from build123d import *

# Parameters (mm, degrees)
F1_DEPTH = 139.7
F2_R     = 6.731
F3_DEPTH = 25.4
F4_R     = 6.985
F5_DEPTH = 25.4
F6_R     = 1.27
F7_R     = 1.27


with BuildPart() as f1:
    # F0 (on Top) → F1 (new body)
    with BuildSketch(Plane.XY):
        Polygon((25.4, 0), (0, 9.525), (-25.4, 0), (0, -9.525), align=None)
    extrude(amount=F1_DEPTH)

    # F2 (on Top) → F3 (join)
    with BuildSketch(Plane.XY):
        Circle(F2_R)
    extrude(amount=-F3_DEPTH)

    # F4 (on face) → F5 (cut)
    with BuildSketch(Plane.XY.offset(139.7)):
        Circle(F4_R)
    extrude(amount=-F5_DEPTH, mode=Mode.SUBTRACT)

    # F6
    f6_edges = [f1.edges().sort_by_distance(p)[0] for p in [
        (-6.985, 0, 114.3),
        (-6.985, 0, 139.7),
    ]]
    fillet(f6_edges, radius=F6_R)

    # F7
    f7_edges = [f1.edges().sort_by_distance(p)[0] for p in [
        (-6.731, 0, -25.4),
        (-6.731, 0, 0),
    ]]
    fillet(f7_edges, radius=F7_R)


solid = f1.part
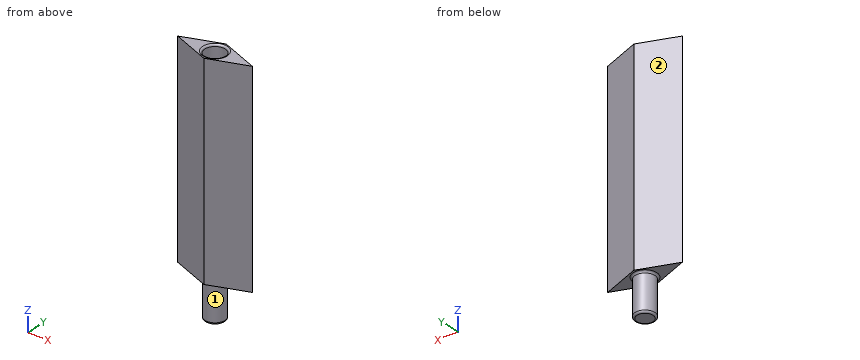
The listing builds one solid part. Answer for the finished solid, in the listing's coordinates (mm). Face numbers are marked on the shaded views. A direction names the side the tool comes from. Coordinates: 2 decimals unless noted, no trailing zeros. Write each loop counter-clockwise with the first axis right and the second up, starting at its lowest first coordinate (ties: lowest second). Pieces come first, ordered by that corner, then holes. Notation, with made-up numbers: (8, -38) - (27, -38) arc R36 ccw to (27, 0) - close; hole circle Ø4 at (11.5, 49.25). An arc over 180 degrees is marked (long way). Return JSON: item names as keys, results as strings.
1. Consider line 1 along Y through (x, z) = (0, 124) (3 decimals); line 2 along Z through (x, y) = (-1.5, 8.25); line 3 along Y through (x, z) = (13, 68). Determine where each line is inside the solid, lowest interval first.
Final values:
{"line 1": "-9.525 to -6.985, 6.985 to 9.525", "line 2": "0 to 139.7", "line 3": "-4.65 to 4.65"}
2. Which of the six approach directions +Z, -Z, +X, -X, +Y, -Y give full straight-line access (tool end or side, diameter ignored) to the marked faces 1 and 2?
Final values:
{"face 1": "-Z", "face 2": "+Z, -Z, -X, +Y"}
3. Each of these flat-tipped pins is pushed along its axis until it touches: pin 1 Ø5 at (x, z) = (15.5, 59) entering from +Y; pin 2 Ø5.5 at (x, y) = (-2, -2) entering from +Z; pin 3 Ø1 at (x, y) = (5, -3.5) entering from -Z. Where does it stop, or does it pass through?
Final values:
{"pin 1": "y = 4.65", "pin 2": "z = 114.3", "pin 3": "z = -25.39"}
4. The part is cut by section A-A on z = 44.5. Determine the outline of the cut face in (x, y) (3 decimals).
Final values:
{"outline": "(-25.4, 0) - (0, -9.525) - (25.4, 0) - (0, 9.525) - close"}
5. The part is cut by section B-B on x = 20.5. Determine the outline of the cut face in (y, z).
Final values:
{"outline": "(-1.84, 0) - (1.84, 0) - (1.84, 139.7) - (-1.84, 139.7) - close"}
